from build123d import *

# Parameters (mm, degrees)
PAD_DEPTH       = 25.4
SKETCH002_R     = 1.75
POCKET001_DEPTH = 16.261


with BuildPart() as part:
    # Sketch → Pad (new body)
    with BuildSketch(Plane.XY):
        with BuildLine():
            Line((-8.13, 0), (0, 0))
            Line((0, 0), (0, 3.45))
            Line((-2.05, 3.45), (0, 3.45))
            Line((-2.05, 15.76), (-2.05, 3.45))
            ThreePointArc((-2.05, 15.76), (-2.533756, 16.259736), (-3.048945, 15.79247))
            Line((-3.048945, 15.79247), (-3.76, 4.86617))
            Line((-3.76, 4.86617), (-4.145, 4.16617))
            ThreePointArc((-6.145, 4.16617), (-5.145, 2.22), (-4.145, 4.16617))
            Line((-6.53, 4.86617), (-6.145, 4.16617))
            Line((-7.130755, 15.787462), (-6.53, 4.86617))
            ThreePointArc((-7.130755, 15.787462), (-7.643736, 16.259811), (-8.13, 15.76))
            Line((-8.13, 0), (-8.13, 15.76))
        make_face()
    pad = extrude(amount=PAD_DEPTH)

    # Mirrored: Pad across Sketch V_Axis
    add(pad.mirror(Plane(origin=(0, 0, 0), x_dir=(0, 0, 1), z_dir=(1, 0, 0))))

    # Sketch002 → Pocket001 (cut, through all)
    with BuildSketch(Plane.XZ):
        with Locations((0, 18.29)):
            Circle(SKETCH002_R)
    extrude(amount=-POCKET001_DEPTH, mode=Mode.SUBTRACT)


solid = part.part
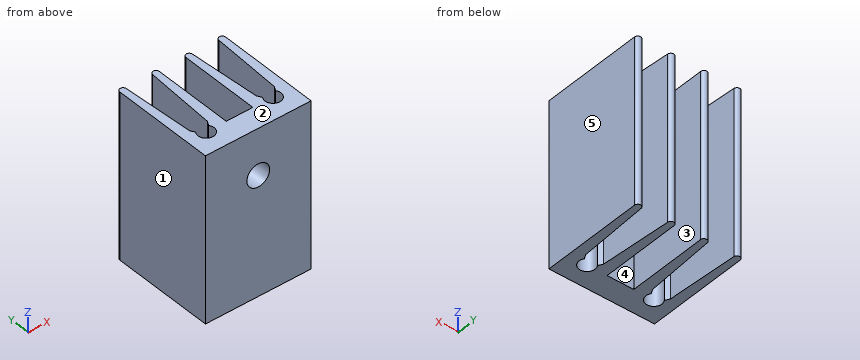
The listing builds one solid part. Answer for the finished solid, in the listing's coordinates (mm). Face numbers are marked on the shaded views. A direction names the side the tool comes from. Coordinates: 2 decimals unless noted, no trailing zeros. Order: outer loops, then holes, each group sorted by start corner. A loop starts at its lowest first (then second) coordinate and runs counter-clockwise, first axis right, second up. Notation, with made-up numbers: (0, 11.25) -> (56, 11.25) arc R19 ccw to (56, 20.25) -> close; hole circle Ø2 at (8, -33.75). An arc over 180 degrees is marked (long way). Answer in a Markdown table with one row per item. Add a question column.
Item 1: Find section B-B (x = -0.5). Write down the section's boundary in (y, z).
Item 2: Find section C-C (z = 17.5). Write down the section's boundary in (x, y) (3 decimals).
Item 3: Find the intervals of material crossed by L1, parallel to X at y = 7.5, z = 2; L2, parallel to X at y = 8.5, z = 2.25; L3, parallel to Z at x = 0, y = 1.2, in increasing order. Write a range as from..to.
Item 4: Find section D-D (z = 5). Write down the section's boundary in (x, y) (3 decimals).
Item 5: Determine the mould class of the marked faces 1, 2 and 3 for opening direction X: +X half, -X half, draft (parallel to the pull), parting line (faces both ways), or undercut.
Item 6: This flat-tipped pin is pushed along its axis until it touches: P1, Ø1, axis at x = -5.5, z = 22, coming from the +Y side. Where does it stop, or does it pass through?
Item 7: Find section A-A (y = 7). Write down the section's boundary in (x, z), then the cut area to 3 significant figures.
Item 8: Which of the six approach directions +Z, -Z, +X, -X, +Y, -Y give full straight-line access (tool end or side, diameter ignored) to the marked faces 4 and 5?
Result set:
| question | item | result |
|---|---|---|
| 1 | outline | (0, 0) -> (3.45, 0) -> (3.45, 16.61) -> (0, 16.61) -> close; (0, 19.97) -> (3.45, 19.97) -> (3.45, 25.4) -> (0, 25.4) -> close |
| 2 | outline | (-8.13, 0) -> (-1.562, 0) -> (-1.562, 3.45) -> (-2.05, 3.45) -> (-2.05, 15.76) arc R0.5 ccw to (-3.049, 15.792) -> (-3.76, 4.866) -> (-4.145, 4.166) arc R1.23 cw (long way) to (-6.145, 4.166) -> (-6.53, 4.866) -> (-7.131, 15.787) arc R0.5 ccw to (-8.13, 15.76) -> close; (1.562, 0) -> (8.13, 0) -> (8.13, 15.76) arc R0.5 ccw to (7.131, 15.787) -> (6.53, 4.866) -> (6.145, 4.166) arc R1.23 cw (long way) to (4.145, 4.166) -> (3.76, 4.866) -> (3.049, 15.792) arc R0.5 ccw to (2.05, 15.76) -> (2.05, 3.45) -> (1.562, 3.45) -> close |
| 3 | L1 | x = -8.13..-6.67, -3.59..-2.05, 2.05..3.59, 6.67..8.13 |
| 3 | L2 | x = -8.13..-6.73, -3.52..-2.05, 2.05..3.52, 6.73..8.13 |
| 3 | L3 | z = 0..16.54, 20.04..25.4 |
| 4 | outline | (-8.13, 0) -> (8.13, 0) -> (8.13, 15.76) arc R0.5 ccw to (7.131, 15.787) -> (6.53, 4.866) -> (6.145, 4.166) arc R1.23 cw (long way) to (4.145, 4.166) -> (3.76, 4.866) -> (3.049, 15.792) arc R0.5 ccw to (2.05, 15.76) -> (2.05, 3.45) -> (-2.05, 3.45) -> (-2.05, 15.76) arc R0.5 ccw to (-3.049, 15.792) -> (-3.76, 4.866) -> (-4.145, 4.166) arc R1.23 cw (long way) to (-6.145, 4.166) -> (-6.53, 4.866) -> (-7.131, 15.787) arc R0.5 ccw to (-8.13, 15.76) -> close |
| 5 | face 1 | -X half |
| 5 | face 2 | draft |
| 5 | face 3 | undercut |
| 6 | P1 | stops at y = 2.57 |
| 7 | outline | (-8.13, 0) -> (-6.65, 0) -> (-6.65, 25.4) -> (-8.13, 25.4) -> close; (-3.62, 0) -> (-2.05, 0) -> (-2.05, 25.4) -> (-3.62, 25.4) -> close; (2.05, 0) -> (3.62, 0) -> (3.62, 25.4) -> (2.05, 25.4) -> close; (6.65, 0) -> (8.13, 0) -> (8.13, 25.4) -> (6.65, 25.4) -> close |
| 7 | area | 155 mm² |
| 8 | face 4 | +Z, -Z, +Y |
| 8 | face 5 | +Z, -Z, +X, +Y, -Y |
